from build123d import *

# Parameters (mm, degrees)
SKETCH153_W      = 176
SKETCH153_H      = 2.5
EXTRUDE139_DEPTH = 4
SKETCH163_R      = 8
SKETCH163_R_2    = 9
EXTRUDE145_DEPTH = 4
SKETCH034_W      = 66
SKETCH034_H      = 49
EXTRUDE028_DEPTH = 4
SKETCH148_W      = 174
SKETCH148_H      = 90
EXTRUDE136_DEPTH = 2


with BuildPart() as clamshell:
    # Sketch153 → Extrude139 (new body)
    with BuildSketch(Plane(origin=(0, 0, 4.32), x_dir=(1, 0, 0), z_dir=(0, 0, -1))):
        with Locations((278, -270.25)):
            Rectangle(SKETCH153_W, SKETCH153_H)
    extrude(amount=-EXTRUDE139_DEPTH)


with BuildPart() as extrude145:
    # Sketch163 → Extrude145 (new body)
    with BuildSketch(Plane(origin=(0, 0, 4.32), x_dir=(1, 0, 0), z_dir=(0, 0, -1))):
        with Locations((206, -202)):
            Circle(SKETCH163_R)
        with Locations((206, -227.431152)):
            Circle(SKETCH163_R)
        with Locations((206, -253)):
            Circle(SKETCH163_R)
        with Locations((343, -200.226852)):
            Circle(SKETCH163_R_2)
        with Locations((343, -227.384705)):
            Circle(SKETCH163_R_2)
        with Locations((343, -251.212372)):
            Circle(SKETCH163_R_2)
        with Locations((245.289581, -196)):
            Circle(SKETCH163_R)
        with Locations((269.509308, -196)):
            Circle(SKETCH163_R)
        with Locations((294.293335, -196)):
            Circle(SKETCH163_R)
    extrude(amount=-EXTRUDE145_DEPTH)


with BuildPart() as bottom_holes:
    # Sketch034 → Extrude028 (new body)
    with BuildSketch(Plane(origin=(0, 0, 4.32), x_dir=(1, 0, 0), z_dir=(0, 0, -1))):
        with Locations((269, -239.5)):
            Rectangle(SKETCH034_W, SKETCH034_H)
    extrude(amount=-EXTRUDE028_DEPTH)

    # Compound007: union clamshell, Extrude145
    add(clamshell.part)
    add(extrude145.part)


with BuildPart() as floor001:
    # Sketch148 → Extrude136 (new body)
    with BuildSketch(Plane(origin=(0, 0, 5.32), x_dir=(1, 0, 0), z_dir=(0, 0, -1))):
        with Locations((278, -225)):
            Rectangle(SKETCH148_W, SKETCH148_H)
    extrude(amount=-EXTRUDE136_DEPTH)

    # Cut008: cut bottom holes
    add(bottom_holes.part, mode=Mode.SUBTRACT)


solid = floor001.part
Model file for the job. Use its own axes, mm. Give positions to 0.01 mm unless a question says otherwise; leave off trailing zeros. Order: outer loops, then holes, each group sorted by start corner. A loop starts at its lowest first (then second) coordinate and runs counter-clockwise, first axis right, second up. Notation, with made-up numbers: (10, -11.5) - (54, -11.5) arc R26 ccw to (54, 19.5) - close; hole circle Ø4 at (23.25, 81.5). An arc over 180 degrees is marked (long way). One line per item, written item: value.
Item 1: Slice it at A-A (x = 206). List the corners of the cut face in (y, z).
Response values:
outline: (180, 5.32) - (194, 5.32) - (194, 7.32) - (180, 7.32) - close; (210, 5.32) - (219.43, 5.32) - (219.43, 7.32) - (210, 7.32) - close; (235.43, 5.32) - (245, 5.32) - (245, 7.32) - (235.43, 7.32) - close; (261, 5.32) - (269, 5.32) - (269, 7.32) - (261, 7.32) - close
Item 2: Slice it at D-D (y = 202). List the corners of the cut face in (x, z).
Response values:
outline: (191, 5.32) - (198, 5.32) - (198, 7.32) - (191, 7.32) - close; (214, 5.32) - (240, 5.32) - (240, 7.32) - (214, 7.32) - close; (250.58, 5.32) - (264.22, 5.32) - (264.22, 7.32) - (250.58, 7.32) - close; (274.8, 5.32) - (289, 5.32) - (289, 7.32) - (274.8, 7.32) - close; (299.58, 5.32) - (334.18, 5.32) - (334.18, 7.32) - (299.58, 7.32) - close; (351.82, 5.32) - (365, 5.32) - (365, 7.32) - (351.82, 7.32) - close
Item 3: Slice it at B-B (y = 248.5). List the corners of the cut face in (x, z).
Response values:
outline: (191, 5.32) - (199.39, 5.32) - (199.39, 7.32) - (191, 7.32) - close; (212.61, 5.32) - (236, 5.32) - (236, 7.32) - (212.61, 7.32) - close; (302, 5.32) - (334.42, 5.32) - (334.42, 7.32) - (302, 7.32) - close; (351.58, 5.32) - (365, 5.32) - (365, 7.32) - (351.58, 7.32) - close
Item 4: Wall check: line 1 (Y direction, x = 206, z = 6.55); line 2 (Y direction, x = 343, z = 6.8); line 3 (Y direction, x = 269.5, z = 7.05). Give the ranges that are in metal, low to high.
Response values:
line 1: 180 to 194, 210 to 219.43, 235.43 to 245, 261 to 269
line 2: 180 to 191.23, 209.23 to 218.38, 236.38 to 242.21, 260.21 to 269
line 3: 180 to 188, 204 to 215, 264 to 269
Item 5: Slice it at C-C (z = 6.05). Give the number of separate pieces and of enclosed holes in the cut face, then the cut area to 3 significant figures.
Response values:
separate pieces: 1
enclosed holes: 10
area: 10,300 mm2
Item 6: Two-plate mould, pull along X, no slides. Class faces 1 (the cylindrical face through (287.945, 200.868, 6.306)), 2 (the flat face through (277, 214, 7.32)): released by +X, released by -X, zero draft, split by the parting line, or undercut.
Response values:
face 1: undercut
face 2: zero draft
